Geometry check sheet. Reference: the model listing, model coordinates, mm. Face numbers are marked on the shaded views. A direction names the side the tool comes from. Give positions to 0.01 mm unless a question says otherwise; leave off trailing zeros. Order: outer loops, then holes, each group sorted by start corner. A loop starts at its lowest first (then second) coordinate and runs counter-clockwise, first axis right, second up. Notation, with made-up numbers: M 45.25,15.25 L 69.25,15.25 A18 cw 69.25,27.25 Z; hole C 17,62 d8. An arc over 180 degrees is marked long. Put each result on its own line as item: value. Start each with the question number.
Q1. Access from +Z, -Z, +X, -X, +Y, -Y to the whole of each face (thin tool, end or side, straight path). Record for the marked faces 1, 2, 3, 4 and 5.
Q2. Mould release check, pull along X, two halves, no side actions. Record for the marked faces 6, 7 and 8: +X half, -X half, draft (parallel to the pull), parting line (faces both ways), or undercut.
Q3. Material ranges on L1, parallel to Z at x = 6, y = -20; L2, parallel to X at y = -30.5, z = 1; L3, parallel to Y at x = -6, z = 0, recorded low to high.
Q4. Section check C-C on x = 0. Record the cut outline in (y, z).
Q5. Go/stop test with flat-tipped pins: pin 1 (1.5 mm diameter, centred on x = -7.5, y = -17.5, fed in from +Z); pin 2 (9 mm diameter, centred on y = -15, z = 4, fed in from -X); pin 3 (4 mm diameter, centred on x = -23.5, z = -3, fed in from -Y); pin 4 (18 mm diameter, centred on x = -11.5, z = 1, fed in from -Y). Record where each tip stops, or that it passes through.
Q6. Section check A-A on y = -20. Record the cut outline in (x, z).
Q7. Section check B-B on z = 0. Record the cut outline in (x, y).
Q8. Section check D-D on x = -24. Record the cut outline in (y, z), then the cut area to 3 significant figures.
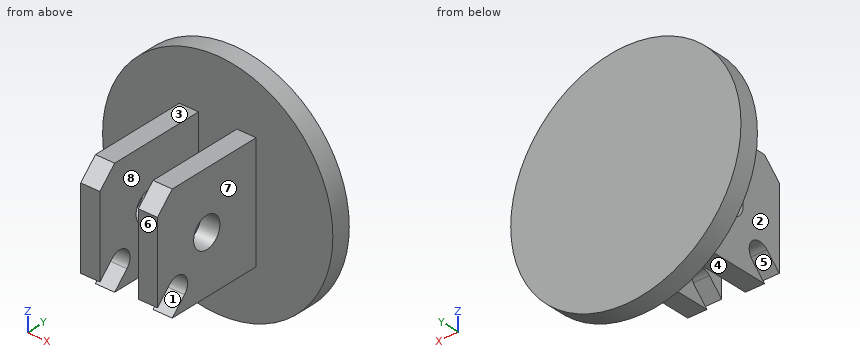
```python
from build123d import *

# Parameters (mm, degrees)
SKETCH001_R  = 30
PAD_DEPTH    = 5
SKETCH_R     = 4
PAD001_DEPTH = 10
SKETCH002_W  = 10
SKETCH002_H  = 30
POCKET_DEPTH = 15


with BuildPart() as part:
    # Sketch001 → Pad (new body)
    with BuildSketch(Plane.XZ):
        Circle(SKETCH001_R)
    extrude(amount=PAD_DEPTH)

    # Sketch → Pad001 (join, symmetric)
    with BuildSketch(Plane.YZ):
        with BuildLine():
            ThreePointArc((-26.774038, -11.264166), (-26.774038, -6.774038), (-31.264166, -6.774038))
            Line((-31.264166, -6.774038), (-35, -10.509872))
            Line((-35, -10.509872), (-35, 10.509872))
            Line((-35, 10.509872), (-30.509872, 15))
            Line((-30.509872, 15), (-0.1, 15))
            Line((-0.1, 15), (-0.1, -15))
            Line((-0.1, -15), (-30.509872, -15))
            Line((-30.509872, -15), (-26.774038, -11.264166))
        make_face()
        with Locations((-20, 0)):
            Circle(SKETCH_R, mode=Mode.SUBTRACT)
    extrude(amount=PAD001_DEPTH, both=True)

    # Sketch002 → Pocket (cut, symmetric)
    with BuildSketch(Plane.XY):
        with Locations((0, -20)):
            Rectangle(SKETCH002_W, SKETCH002_H)
    extrude(amount=POCKET_DEPTH, both=True, mode=Mode.SUBTRACT)


solid = part.part
```
Results found:
1. face 1: +X, -X, -Y
1. face 2: +Z, -Z, -X, -Y
1. face 3: +Z, +X, -X, -Y
1. face 4: -Z, +X, -X, -Y
1. face 5: -Z, +X, -X
2. face 6: draft
2. face 7: +X half
2. face 8: undercut
3. L1: z = -15 to -4, 4 to 15
3. L2: x = -10 to -5, 5 to 10
3. L3: y = -35 to -24, -16 to 0
4. outline: M -5,-30 L 0,-30 L 0,30 L -5,30 Z
5. pin 1: stops at z = 15
5. pin 2: stops at x = -10
5. pin 3: stops at y = -5
5. pin 4: stops at y = -35
6. outline: M -10,-15 L -5,-15 L -5,-4 L -10,-4 Z; M -10,4 L -5,4 L -5,15 L -10,15 Z; M 5,-15 L 10,-15 L 10,-4 L 5,-4 Z; M 5,4 L 10,4 L 10,15 L 5,15 Z
7. outline: M -30,-5 L -10,-5 L -10,-16 L -5,-16 L -5,-5 L 5,-5 L 5,-16 L 10,-16 L 10,-5 L 30,-5 L 30,0 L -30,0 Z; M -10,-35 L -5,-35 L -5,-24 L -10,-24 Z; M 5,-35 L 10,-35 L 10,-24 L 5,-24 Z
8. outline: M -5,-18 L 0,-18 L 0,18 L -5,18 Z
8. area: 180 mm^2
